Check sheet for the modelled part. Datum: model origin and axes. Units: mm. A direction names the side the tool comes from. Round coordinates to 2 decimals unless told otherwise and drop trailing zeros. Write each loop counter-clockwise with the first axis right and the second up, starting at its lowest first coordinate (ties: lowest second). Pieces come first, ordered by that corner, then holes. Notation, with made-up numbers: (27, 51.25) -> (74, 51.25) arc R19 cw to (74, 83.25) -> close; hole circle Ø1 at (65, 45.5). An arc over 180 degrees is marked (long way). Put each result on its own line as item: value. Start each with the question number.
Autodesk Fusion 360 part; units mm, degrees
sketch "Sketch1" plane through (0, 0, 0) normal (0, 0, 1) x (1, 0, 0)
  circle A0 centre (0, 0) radius 10
  circle A1 centre (0, 0) radius 3.5
  line L0 (0, 3.5) -> (0, -2.5)
  line L1 (0, -2.5) -> (2.4495, -2.5)
  line L2 (0, -2.5) -> (-2.4495, -2.5)
  circle A2 centre (0, 0) radius 7.5
  dimension "d1" = 20
  dimension "d2" = 7
extrude "Extrude1" add sketch "Sketch1" along normal blind 12 contours A0 | A1 L0 L1 | A1 L0 L2 | A1 L1 L2 | A2
extrude "Extrude2" cut sketch "Sketch1" along normal blind 10 contours A1 L0 L1 | A1 L0 L2
sketch "Sketch2" plane through (0, 0, 0) normal (0, 0, 1) x (1, 0, 0)
extrude "Extrude3" cut 1 faces at (2.3712, -3.5556, 12) along direction (0, 0, -1) blind 1
extrude "Extrude4" add sketch "Sketch1" against normal blind 3.5 contours A0
1. Section check A-A, the plane x = 6. Enter the section's corners in (y, z).
2. Draft check along Y on faces 1 (the flat face through (0, -2.5, 5)), 2 (the flat face through (0, 0, 11)), 3 (the cylindrical face through (-2.17, -9.76, 3.85)). Enter one of: released by +Y, released by -Y, zero draft, split by the parting line, or undercut.
3. Section check B-B, the plane z = 5. Enter the section's corners in (x, y).
4. Material ranges on L1, parallel to Y at x = 0, z = 4.5; L2, parallel to Y at x = 0, z = -0.8; L3, parallel to X at y = 1, z = 4, recorded low to high. Write a range as [from, to].
5. Gauge pin test, flat ends, axial feed: P1, Ø5.5, axis at x = 0, y = 0, coming from the -Z side; P2, Ø1.5, axis at x = -8, z = 9, coming from the +Y side; P3, Ø4, axis at x = 7, z = 3, coming from the +Y side. Record the tip position at first contact, or that the pin passes through.
6. Section check D-D, the plane x = 0. Enter the section's corners in (y, z), then the cut area to 4 significant figures.
7. Access from +Z, -Z, +X, -X, +Y, -Y to the whole of each face (thin tool, end or side, straight path). Record for faces 4 (the flat face through (4, 7, -3.5)), 5 (the cylindrical face through (-7.493, 0.33, -1.726)).
8. Section check C-C, the plane y = 0. Enter the section's corners in (x, z).
Reply:
1. outline: (-8, -3.5) -> (-4.5, -3.5) -> (-4.5, 0) -> (4.5, 0) -> (4.5, -3.5) -> (8, -3.5) -> (8, 11) -> (-8, 11) -> close
2. face 1: undercut
2. face 2: zero draft
2. face 3: split by the parting line
3. outline: circle Ø20 at (0, 0); hole (-2.45, -2.5) -> (2.45, -2.5) arc R3.5 ccw (long way) to start
4. L1: y = [-10, -2.5], [3.5, 10]
4. L2: y = [-10, -7.5], [7.5, 10]
4. L3: x = [-9.95, -3.35], [3.35, 9.95]
5. P1: stops at z = 0
5. P2: stops at y = 6.89
5. P3: stops at y = 8.66
6. outline: (-10, -3.5) -> (-7.5, -3.5) -> (-7.5, 0) -> (-2.5, 0) -> (-2.5, 10) -> (3.5, 10) -> (3.5, 0) -> (7.5, 0) -> (7.5, -3.5) -> (10, -3.5) -> (10, 11) -> (-10, 11) -> close
6. area: 177.5 mm2
7. face 4: -Z, +X, -X, +Y, -Y
7. face 5: -Z
8. outline: (-10, -3.5) -> (-7.5, -3.5) -> (-7.5, 0) -> (-3.5, 0) -> (-3.5, 10) -> (3.5, 10) -> (3.5, 0) -> (7.5, 0) -> (7.5, -3.5) -> (10, -3.5) -> (10, 11) -> (-10, 11) -> close
